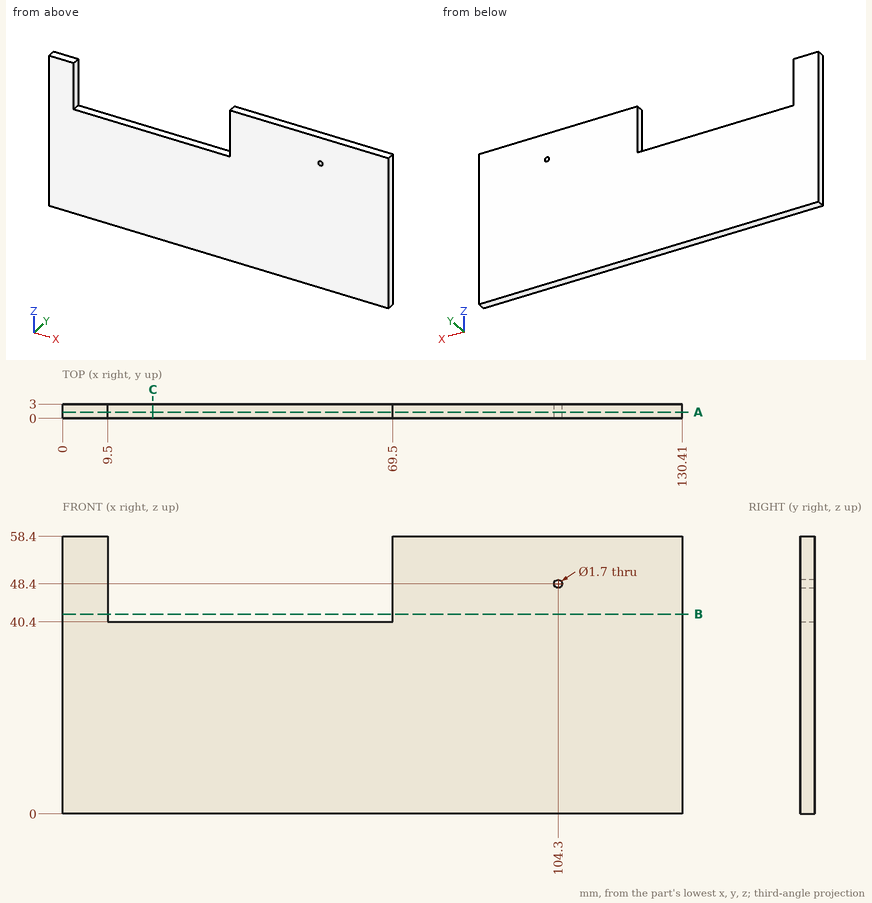
Geometry check sheet. Reference: drawing and pictorial views, mm from the part's lowest x, y, z. Coordinates: 2 decimals unless noted, no trailing zeros. Write each loop counter-clockwise with the first axis right and the second up, starting at its lowest first coordinate (ties: lowest second). Pieces come first, ordered by that corner, then holes. Notation, with made-up numbers: (79.5, -7) -> (98.5, -7) arc R13 ccw to (98.5, 18) -> close; hole circle Ø8 at (35.25, 71). An arc over 180 degrees is marked (long way). One line per question, with ' | ' between items.
1. Cross-section at C-C on x = 19. Record the cut outline in (y, z).
Answers:
outline: (0, 0) -> (3, 0) -> (3, 40.4) -> (0, 40.4) -> close
2. Depth check by flat-ended pin: pin 1 Ø1.5 at (x, y) = (27, 1.5) entering from +Z. Enter the tip coordinate at first touch or a pass-through.
Answers:
pin 1: stops at z = 40.4
3. Thickness scan on probe 1 along X at (y, z) = (1.85, 48.4); probe 2 along Z at (x, y) = (104.3, 0.75); probe 3 along X at (y, z) = (1.6, 46). Record the ranges inside material, lowest first. Write a range as from..to.
Answers:
probe 1: x = 0..9.5, 69.5..103.45, 105.15..130.41 | probe 2: z = 0..47.55, 49.25..58.4 | probe 3: x = 0..9.5, 69.5..130.41
4. Cross-section at B-B on z = 42. Record the cut outline in (x, y).
Answers:
outline: (0, 0) -> (9.5, 0) -> (9.5, 3) -> (0, 3) -> close; (69.5, 0) -> (130.41, 0) -> (130.41, 3) -> (69.5, 3) -> close
5. Cross-section at A-A on y = 1.3. Record the cut outline in (x, z).
Answers:
outline: (0, 0) -> (130.41, 0) -> (130.41, 58.4) -> (69.5, 58.4) -> (69.5, 40.4) -> (9.5, 40.4) -> (9.5, 58.4) -> (0, 58.4) -> close; hole circle Ø1.7 at (104.3, 48.4)
